For this review, use the dimensioned drawing (mm, ordinates from the lowest corner) and the shaded views. A direction names the side the tool comes from. Coordinates: 2 decimals unless noted, no trailing zeros. Loops run counter-clockwise (first coordinate to the right, second up) from the corner with the lowest first, then second, coordinate; pieces in that order, holes last. Notation, with made-up numbers: (-27, -33.5) -> (-9, -33.5) arc R6 cw to (-9, -22.5) -> close; hole circle Ø7 at (-23, 49.25). An arc over 180 degrees is marked (long way). Answer as a JSON object with one key per item and string values.
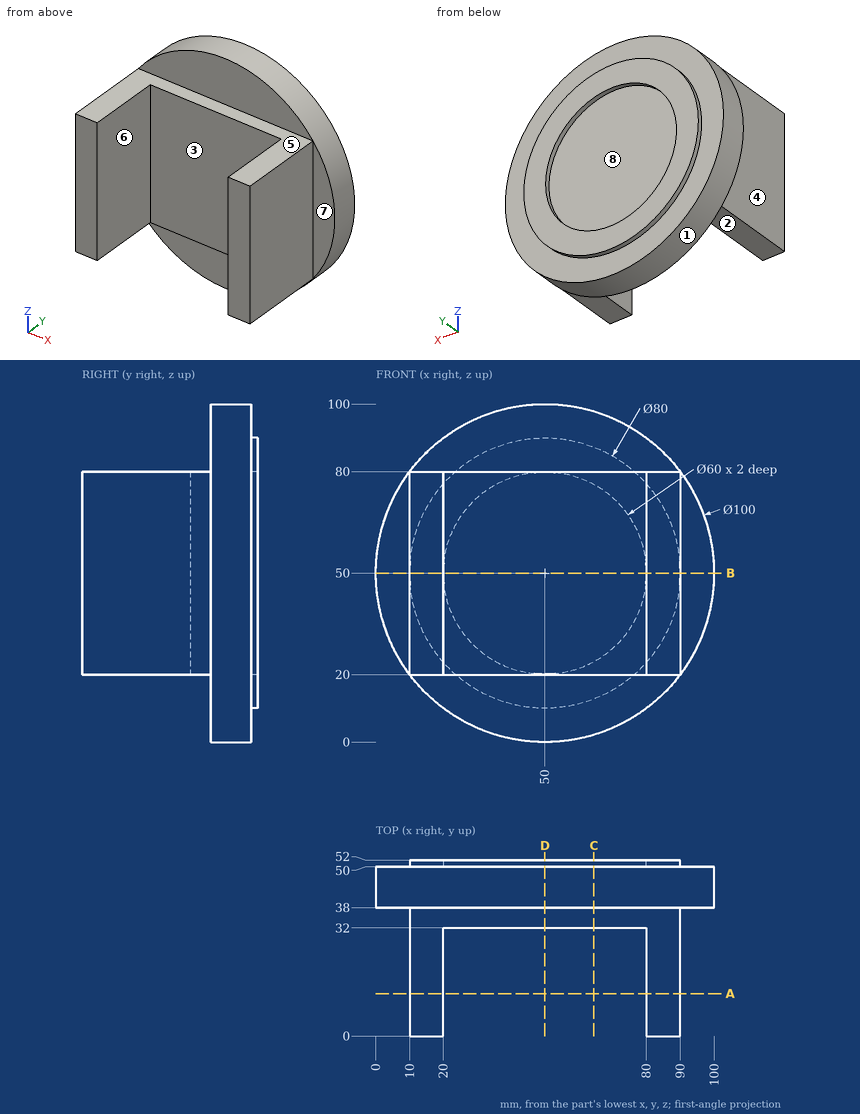
1) Add section B-B, the plane z = 50. Give the boundary of the cut face in (x, y), and give its area (3 significant figures).
Completed:
{"outline": "(0, 38) -> (10, 38) -> (10, 0) -> (20, 0) -> (20, 32) -> (80, 32) -> (80, 0) -> (90, 0) -> (90, 38) -> (100, 38) -> (100, 50) -> (90, 50) -> (90, 52) -> (80, 52) -> (80, 50) -> (20, 50) -> (20, 52) -> (10, 52) -> (10, 50) -> (0, 50) -> close", "area": "2,360 mm²"}
2) For the marked faces 5, 6, 7 and 8, list the 3-axis set-ups (+Z, -Z, +X, -X, +Y, -Y) from which the entire face can be reached by the end or side of a thin tool; tool diameter is ignored.
Completed:
{"face 5": "+Z, +X, -X, -Y", "face 6": "+Z, -Z, -Y", "face 7": "+Z, -Z, +X, -Y", "face 8": "+Y"}
3) Add section C-C, the plane x = 64.5. Give the boundary of the cut face in (y, z), and give its area (3 significant figures).
Completed:
{"outline": "(32, 20) -> (38, 20) -> (38, 2.15) -> (50, 2.15) -> (50, 12.72) -> (52, 12.72) -> (52, 23.74) -> (50, 23.74) -> (50, 76.26) -> (52, 76.26) -> (52, 87.28) -> (50, 87.28) -> (50, 97.85) -> (38, 97.85) -> (38, 80) -> (32, 80) -> close", "area": "1,550 mm²"}
4) Wall thickness on probe 1 along Z at (x, y) = (50, 51); probe 2 along Y at (x, z) = (64.5, 69): over which ranges is each line inside the solid? List them lowest first.
Completed:
{"probe 1": "10 to 20, 80 to 90", "probe 2": "32 to 50"}
5) Add section D-D, the plane x = 50. Give the boundary of the cut face in (y, z), and give its area (3 significant figures).
Completed:
{"outline": "(32, 20) -> (38, 20) -> (38, 0) -> (50, 0) -> (50, 10) -> (52, 10) -> (52, 20) -> (50, 20) -> (50, 80) -> (52, 80) -> (52, 90) -> (50, 90) -> (50, 100) -> (38, 100) -> (38, 80) -> (32, 80) -> close", "area": "1,600 mm²"}
6) Clearance check with flat-ended pins moving along their axes: pin 1 Ø19 at (x, y) = (67, 19) entering from +Z; pin 2 Ø3 at (x, y) = (20.5, 31.5) entering from +Z; pin 3 Ø8 at (y, z) = (37, 70.5) entering from -X; pin 4 Ø6 at (x, z) = (35, 95) entering from -Y. State where each tip first meets the part, or that it passes through.
Completed:
{"pin 1": "through", "pin 2": "z = 80", "pin 3": "x = 2.85", "pin 4": "y = 38"}
7) Add section A-A, the plane y = 12.5. Give the boundary of the cut face in (x, z).
Completed:
{"outline": "(10, 20) -> (20, 20) -> (20, 80) -> (10, 80) -> close; (80, 20) -> (90, 20) -> (90, 80) -> (80, 80) -> close"}
8) The part is to be moulded in two halves that separate along X. For the marked faces 1, 2, 3 and 4, say which applies: pulls with the +X half, pulls with the -X half, needs draft (parallel to the pull), parting line crosses it, or undercut.
Completed:
{"face 1": "parting line crosses it", "face 2": "needs draft", "face 3": "undercut", "face 4": "pulls with the -X half"}
